Input: part model. Units: mm. Frame: model coordinates. A direction names the side the tool comes from. Round coordinates to 2 decimals unless told otherwise and drop trailing zeros. Loops run counter-clockwise (first coordinate to the right, second up) from the corner with the lowest first, then second, coordinate; pieces in that order, holes last. Notation, with made-up numbers: M 67,-1 L 114,-1 A22 cw 114,16 Z; hole C 56.25,71.25 d8. An arc over 180 degrees is marked long. Put each result on its own line as item: value. Start each with the question number.
1) Pin query (flat end, axial travel): pin 1 (3 mm diameter, centred on x = -25, z = 63, fed in from +Y); pin 2 (1.9 mm diameter, centred on x = -24.5, y = 244, fed in from +Z); pin 3 (1.5 mm diameter, centred on y = 239, z = 21.5, fed in from -X); pin 4 (1 mm diameter, centred on y = 234, z = 42.5, fed in from -X). Return the tip coordinate at first contact, or that it passes through.
2) Reachability of faces 5 (the face through (-25, 248, 22.596)), 6 (the face through (-31.011, 233.11, 82.827)), 7 (the face through (-34.875, 263, 52)) from +Z, -Z, +X, -X, +Y, -Y: full face, straight path, thin tool, end or side. Return the list, or none.
3) Line query: probe 1 along X at (y, z) = (230, 34); probe 2 along Z at (x, y) = (-26.5, 238); probe 3 along Y at (x, z) = (-32.75, 81). Output: solid intervals per line, ascending.
4) Section B-B on y = 227.5. Output: boundary loops of the cut face in (x, z).
5) Section C-C on y = 240.5. Output: boundary loops of the cut face in (x, z).
6) Section D-D on z = 32. Output: boundary loops of the cut face in (x, y).
7) Section A-A on z = 57.5. Output: boundary loops of the cut face in (x, y).
8) Draft query along Y for faces 1 (the face through (-31.011, 234.075, 52.313)), 2 (the face through (-34.875, 263, 81)), 3 (the face through (-27, 222.383, 39)), 4 (the face through (-31.011, 263.868, 53.246)). Return one class per face: +Y half, -Y half, draft (parallel to the pull), parting line (faces both ways), or undercut.
from build123d import *

# Parameters (mm, degrees)
BOSS_EXTRUDE1_DEPTH = 50.8
SKETCH2_R           = 1.397
BOSS_EXTRUDE3_DEPTH = 7.62
SKETCH4_W           = 25.11
SKETCH4_H           = 28.65
CUT_EXTRUDE2_DEPTH  = 8.846923164


with BuildPart() as part:
    # Sketch1 → Boss-Extrude1 (new body)
    with BuildSketch(Plane(origin=(0, 273.183078415, 0), x_dir=(1, 0, 0), z_dir=(0, 1, 0))):
        with BuildLine():
            Line((-29.667642961, -22.342314993), (-29.667642961, -22.596314993))
            Line((-29.667642961, -22.596314993), (-27.254642961, -22.596314993))
            Line((-27.254642961, -22.596314993), (-27.254642961, -86.096314993))
            Line((-27.254642961, -86.096314993), (-25.984642961, -86.096314993))
            Line((-25.984642961, -86.096314993), (-25.984642961, -22.596314993))
            Line((-25.984642961, -22.596314993), (-23.571642961, -22.596314993))
            Line((-23.571642961, -22.596314993), (-23.571642961, -22.342314993))
            Line((-23.571642961, -22.342314993), (-23.571642961, -19.548314993))
            Line((-23.571642961, -19.548314993), (-19.788719797, -19.548314993))
            ThreePointArc((-19.788719797, -19.548314993), (-19.436721695, -19.313117381), (-19.519312114, -18.897907309))
            Line((-19.519312114, -18.897907309), (-23.406350532, -15.010868891))
            ThreePointArc((-23.406350532, -15.010868891), (-24.147982307, -14.515326382), (-25.022796633, -14.341314993))
            Line((-25.022796633, -14.341314993), (-28.216489288, -14.341314993))
            ThreePointArc((-28.216489288, -14.341314993), (-29.091303615, -14.515326382), (-29.83293539, -15.010868891))
            Line((-29.83293539, -15.010868891), (-33.719973808, -18.897907309))
            ThreePointArc((-33.719973808, -18.897907309), (-33.802564226, -19.313117381), (-33.450566125, -19.548314993))
            Line((-33.450566125, -19.548314993), (-29.667642961, -19.548314993))
            Line((-29.667642961, -19.548314993), (-29.667642961, -22.342314993))
        make_face()
    extrude(amount=-BOSS_EXTRUDE1_DEPTH)

    # Sketch2 → Boss-Extrude3 (add)
    with BuildSketch(Plane.ZY.offset(27.254642961)):
        with Locations((52.494743656, 232.690269259)):
            Circle(SKETCH2_R)
        with Locations((52.494743656, 262.690269259)):
            Circle(SKETCH2_R)
        with Locations((81.494743656, 262.690269259)):
            Circle(SKETCH2_R)
        with Locations((81.494743656, 232.690269259)):
            Circle(SKETCH2_R)
    extrude(amount=BOSS_EXTRUDE3_DEPTH)

    # Sketch4 → Cut-Extrude2 (cut, through all)
    with BuildSketch(Plane.ZY.offset(27.254642961)):
        with Locations((66.994743656, 247.690269259)):
            Rectangle(SKETCH4_W, SKETCH4_H)
    extrude(amount=-CUT_EXTRUDE2_DEPTH, mode=Mode.SUBTRACT)


solid = part.part
Geometry results:
1. pin 1: stops at y = 273.18
1. pin 2: stops at z = 22.6
1. pin 3: stops at x = -29.67
1. pin 4: stops at x = -27.25
2. face 5: +Z, +X, +Y, -Y
2. face 6: -X
2. face 7: +Z, -Z, -X, +Y, -Y
3. probe 1: x = -27.25 to -25.98
3. probe 2: z = 14.34 to 54.44, 79.55 to 86.1
3. probe 3: y = 231.38 to 234, 261.38 to 264
4. outline: M -33.72,18.9 L -29.83,15.01 A2.29 ccw -28.22,14.34 L -25.02,14.34 A2.29 ccw -23.41,15.01 L -19.52,18.9 A0.38 ccw -19.79,19.55 L -23.57,19.55 L -23.57,22.6 L -25.98,22.6 L -25.98,86.1 L -27.25,86.1 L -27.25,22.6 L -29.67,22.6 L -29.67,19.55 L -33.45,19.55 A0.38 ccw Z
5. outline: M -33.72,18.9 L -29.83,15.01 A2.29 ccw -28.22,14.34 L -25.02,14.34 A2.29 ccw -23.41,15.01 L -19.52,18.9 A0.38 ccw -19.79,19.55 L -23.57,19.55 L -23.57,22.6 L -25.98,22.6 L -25.98,54.44 L -27.25,54.44 L -27.25,22.6 L -29.67,22.6 L -29.67,19.55 L -33.45,19.55 A0.38 ccw Z; M -27.25,79.55 L -25.98,79.55 L -25.98,86.1 L -27.25,86.1 Z
6. outline: M -27.25,222.38 L -25.98,222.38 L -25.98,273.18 L -27.25,273.18 Z
7. outline: M -27.25,222.38 L -25.98,222.38 L -25.98,233.37 L -27.25,233.37 Z; M -27.25,262.02 L -25.98,262.02 L -25.98,273.18 L -27.25,273.18 Z
8. face 1: undercut
8. face 2: draft
8. face 3: -Y half
8. face 4: undercut
